For this review, take the finished solid that the model builds, in its own axes (mm). A direction names the side the tool comes from. Give positions to 0.01 mm unless a question says otherwise; leave off trailing zeros. Loops run counter-clockwise (first coordinate to the right, second up) from the corner with the lowest first, then second, coordinate; pieces in that order, holes last. Notation, with made-up numbers: (8, -6.5) -> (19, -6.5) arc R19 cw to (19, 9.5) -> close; hole circle Ø3 at (-22, 83). An arc over 180 degrees is marked (long way). One line per question, with ' | ' between items. Start each with the question number.
(1) Consider section A-A (x = -10.75). Write out the cut boundary in (y, z), and give its area (3 significant figures).
(2) Tool access review of faces 1 (the flat face through (-12.5, -1, -1)), 2 (the flat face through (0.175, -17.864, 9.3)): name each direction out of +Z, -Z, +X, -X, +Y, -Y from which nothing blocks a thin tool from reaching the whole face with its end or side.
(3) Consider section C-C (x = -5.5). Write out the cut boundary in (y, z).
(4) Insertion check: P1, Ø1.5, axis at x = -8.5, y = 30, coming from the +Z side; P2, Ø3, axis at x = -4.5, z = -29.5, coming from the +Y side; P3, Ø6, axis at y = 3, z = 24.5, coming from the +X side; P4, Ø4, axis at x = -8, y = 4.5, coming from the +Z side. Each pin has a flat end and moves straight along its axis. Give the tip position at first contact, or say it passes through.
(5) Wall thickness on probe 1 along Y at (x, z) = (-6.5, -6); probe 2 along Y at (x, z) = (-9, -6); probe 3 along Z at (x, y) = (-7.75, -8): over which ranges is each line inside the solid? List them lowest first.
(6) Draft analysis for pull direction Y (two halves, no side actions). For faces 3 (the cylindrical face through (0, -10, 0)), 4 (the flat face through (12.5, -1, -8)), 5 (the cylindrical face through (-11.02, -1.76, -39.96)), 6 (the flat face through (0.175, 9.17, -17.616)), state which applies: +Y half, -Y half, draft (parallel to the pull), parting line (faces both ways), or undercut.
(7) Consider section B-B (x = 5.25). Write out the cut boundary in (y, z).
from build123d import *

# Parameters (mm, degrees)
CUT_EXTRUDE1_DEPTH               = 62.846584384
F_2_05_2_08_DIAMETER_HOLE1_D     = 2.08
F_2_05_2_08_DIAMETER_HOLE1_DEPTH = 20
F_2_05_2_08_DIAMETER_HOLE1_TIP   = 0.624895044


with BuildPart() as part:
    # Sketch1 → Revolve1 (revolve)
    with BuildSketch(Plane(origin=(0, 0, 0), x_dir=(1, 0, 0), z_dir=(0, 1, 0)), mode=Mode.PRIVATE) as revolve1_sk:
        with BuildLine():
            Line((-12.5, 0), (12.5, 0))
            Line((12.5, 0), (12.5, 40))
            Line((12.5, 40), (9.5, 40))
            ThreePointArc((9.5, 40), (0, 37.599715907), (-9.5, 40))
            Line((-9.5, 40), (-12.5, 40))
            Line((-12.5, 40), (-12.5, 0))
        make_face()
    revolve(revolve1_sk.sketch.rotate(Axis((-12.5, 0, 0), (1, 0, 0)), 180), axis=Axis((-12.5, 0, 0), (1, 0, 0)))

    # Sketch2 → Cut-Extrude1 (cut, through all)
    with BuildSketch(Plane(origin=(12.5, 0, 0), x_dir=(0, 0, -1), z_dir=(1, 0, 0))):
        with BuildLine():
            Line((-4.617486132, 8.870108332), (-13.852458397, 26.610324995))
            ThreePointArc((-13.852458397, 26.610324995), (0, 30), (13.852458397, 26.610324995))
            Line((13.852458397, 26.610324995), (4.617486132, 8.870108332))
            ThreePointArc((4.617486132, 8.870108332), (0, 10), (-4.617486132, 8.870108332))
        make_face()
        with BuildLine():
            Line((26.610324995, -13.852458397), (8.870108332, -4.617486132))
            ThreePointArc((8.870108332, -4.617486132), (10, 0), (8.870108332, 4.617486132))
            Line((8.870108332, 4.617486132), (26.610324995, 13.852458397))
            ThreePointArc((26.610324995, 13.852458397), (30, 0), (26.610324995, -13.852458397))
        make_face()
        with BuildLine():
            Line((-13.852458397, -26.610324995), (-4.617486132, -8.870108332))
            ThreePointArc((-4.617486132, -8.870108332), (0, -10), (4.617486132, -8.870108332))
            Line((4.617486132, -8.870108332), (13.852458397, -26.610324995))
            ThreePointArc((13.852458397, -26.610324995), (0, -30), (-13.852458397, -26.610324995))
        make_face()
        with BuildLine():
            Line((-26.610324995, 13.852458397), (-8.870108332, 4.617486132))
            ThreePointArc((-8.870108332, 4.617486132), (-10, 0), (-8.870108332, -4.617486132))
            Line((-8.870108332, -4.617486132), (-26.610324995, -13.852458397))
            ThreePointArc((-26.610324995, -13.852458397), (-30, 0), (-26.610324995, 13.852458397))
        make_face()
    extrude(amount=-CUT_EXTRUDE1_DEPTH, mode=Mode.SUBTRACT)

    # Ø2.05 (2.08) Diameter Hole1
    with Locations(Plane(origin=(12.5, 0, 0), x_dir=(0, 0, -1), z_dir=(1, 0, 0))):
        with Locations((0, 0)):
            Hole(F_2_05_2_08_DIAMETER_HOLE1_D / 2, depth=F_2_05_2_08_DIAMETER_HOLE1_DEPTH)
            with Locations((0, 0, -(F_2_05_2_08_DIAMETER_HOLE1_DEPTH + F_2_05_2_08_DIAMETER_HOLE1_TIP / 2))):  # 118° drill point
                Cone(0, F_2_05_2_08_DIAMETER_HOLE1_D / 2, F_2_05_2_08_DIAMETER_HOLE1_TIP, mode=Mode.SUBTRACT)


solid = part.part
A:
1) outline: circle Ø80 at (0, 0); hole (-26.61, -13.85) -> (-8.87, -4.62) arc R10 cw to (-8.87, 4.62) -> (-26.61, 13.85) arc R30 ccw to start; hole (-13.85, -26.61) arc R30 ccw to (13.85, -26.61) -> (4.62, -8.87) arc R10 cw to (-4.62, -8.87) -> close; hole (-13.85, 26.61) -> (-4.62, 8.87) arc R10 cw to (4.62, 8.87) -> (13.85, 26.61) arc R30 ccw to start; hole (8.87, -4.62) -> (26.61, -13.85) arc R30 ccw to (26.61, 13.85) -> (8.87, 4.62) arc R10 cw to start | area: 3,490 mm^2
2) face 1: +Z, -Z, -X, +Y, -Y | face 2: +X, -X
3) outline: circle Ø76.74 at (0, 0); hole (-26.61, -13.85) -> (-8.87, -4.62) arc R10 cw to (-8.87, 4.62) -> (-26.61, 13.85) arc R30 ccw to start; hole (-13.85, -26.61) arc R30 ccw to (13.85, -26.61) -> (4.62, -8.87) arc R10 cw to (-4.62, -8.87) -> close; hole (-13.85, 26.61) -> (-4.62, 8.87) arc R10 cw to (4.62, 8.87) -> (13.85, 26.61) arc R30 ccw to start; hole circle Ø2.08 at (0, 0); hole (8.87, -4.62) -> (26.61, -13.85) arc R30 ccw to (26.61, 13.85) -> (8.87, 4.62) arc R10 cw to start
4) P1: stops at z = 26.7 | P2: stops at y = 25.94 | P3: passes through | P4: stops at z = 39.87
5) probe 1: y = -38.22 to -29.39, -11.53 to 11.53, 29.39 to 38.22 | probe 2: y = -39.28 to -29.39, -11.53 to 11.53, 29.39 to 39.28 | probe 3: z = -38.34 to -28.91, -15.37 to 15.37, 28.91 to 38.34
6) face 3: undercut | face 4: draft | face 5: parting line | face 6: undercut
7) outline: circle Ø76.6 at (0, 0); hole (-26.61, -13.85) -> (-8.87, -4.62) arc R10 cw to (-8.87, 4.62) -> (-26.61, 13.85) arc R30 ccw to start; hole (-13.85, -26.61) arc R30 ccw to (13.85, -26.61) -> (4.62, -8.87) arc R10 cw to (-4.62, -8.87) -> close; hole (-13.85, 26.61) -> (-4.62, 8.87) arc R10 cw to (4.62, 8.87) -> (13.85, 26.61) arc R30 ccw to start; hole circle Ø2.08 at (0, 0); hole (8.87, -4.62) -> (26.61, -13.85) arc R30 ccw to (26.61, 13.85) -> (8.87, 4.62) arc R10 cw to start
